from build123d import *

# Parameters (mm, degrees)
F0_W     = 42
F0_H     = 60
F0_R     = 5.1
F1_DEPTH = 25
F2_R     = 8.75
F2_R_2   = 5.1
F3_DEPTH = 35
F4_DEPTH = 60


with BuildPart() as f1:
    # F0 (on Top) → F1 (new body)
    with BuildSketch(Plane.XY):
        with Locations((-21, -12.544838)):
            Rectangle(F0_W, F0_H)
        with Locations((-12, 5.455162)):
            Circle(F0_R, mode=Mode.SUBTRACT)
    extrude(amount=F1_DEPTH)

    # F2 (on face) → F3 (cut)
    with BuildSketch(Plane(origin=(0, 17.455162, 0), x_dir=(-1, 0, 0), z_dir=(0, 1, 0))):
        with Locations((30, 12.5)):
            Circle(F2_R)
        with Locations((30, 12.5)):
            Circle(F2_R_2, mode=Mode.SUBTRACT)
    extrude(amount=-F3_DEPTH, mode=Mode.SUBTRACT)

    # F2 (on face) → F4 (cut)
    with BuildSketch(Plane(origin=(0, 17.455162, 0), x_dir=(-1, 0, 0), z_dir=(0, 1, 0))):
        with Locations((30, 12.5)):
            Circle(F2_R_2)
    extrude(amount=-F4_DEPTH, mode=Mode.SUBTRACT)


solid = f1.part
Could you check a few things on this model? Use its own coordinates, in mm. A direction names the side the tool comes from. Give positions to 0.01 mm unless a question says otherwise; leave off trailing zeros. Loops run counter-clockwise (first coordinate to the right, second up) from the corner with the lowest first, then second, coordinate; pieces in that order, holes last. Notation, with made-up numbers: M 11.5,42.25 L 54.5,42.25 A10 cw 54.5,61.25 Z; hole C -14,69 d8. An arc over 180 degrees is marked long. Answer as a JSON object with one key per item and string values.
Q1. If I drill on probe 1 along Z at (x, y) = (-30, -4); probe 2 along Y at (x, z) = (-12, 12.75); probe 3 along X at (y, z) = (9.5, 17.25), over which ranges is the centre line in solid material (lowest first)? Write a range as [from, to].
Values found:
{"probe 1": "z = [0, 3.75], [21.25, 25]", "probe 2": "y = [-42.54, 0.36], [10.56, 17.46]", "probe 3": "x = [-42, -37.35], [-22.65, -15.11], [-8.89, 0]"}
Q2. If we mould it in two halves opening along X, with no side actions, what happens to faces 1 (the flat face through (0, -13, 12)), 2 (the flat face through (-21, -42.545, 12)), 3 (the cylindrical face through (-7.29, 3.5, 12.32))? For each: pulls with the +X half, pulls with the -X half, needs draft (parallel to the pull), parting line crosses it, or undercut.
Values found:
{"face 1": "pulls with the +X half", "face 2": "needs draft", "face 3": "undercut"}
Q3. Suppose I cut it at A-A, the plane z = 12.5. List the corners of the cut face in (x, y) for me.
Values found:
{"outline": "M -42,-42.54 L -35.1,-42.54 L -35.1,-17.54 L -38.75,-17.54 L -38.75,17.46 L -42,17.46 Z; M -24.9,-42.54 L 0,-42.54 L 0,17.46 L -21.25,17.46 L -21.25,-17.54 L -24.9,-17.54 Z; hole C -12,5.46 d10.2"}
Q4. Suppose I cut it at C-C, the plane z = 20.5. List the corners of the cut face in (x, y) for me, plus the area to 3 significant figures.
Values found:
{"outline": "M -42,-42.54 L 0,-42.54 L 0,17.46 L -26.46,17.46 L -26.46,-17.54 L -33.54,-17.54 L -33.54,17.46 L -42,17.46 Z; hole C -12,5.46 d10.2", "area": "2,190 mm²"}
Q5. For faces 4 (the flat face through (-21, -12, 0)), 5 (the cylindrical face through (-28.861, 0.2, 21.176)), which set-ups out of +Z, -Z, +X, -X, +Y, -Y let a thin tool reach every point of the face, with its end or its side?
Values found:
{"face 4": "-Z, +X, -X, +Y, -Y", "face 5": "+Y"}
Q6. For P1, Ø14, axis at x = -30, z = 12.5, coming from the +Y side, with a flat end and sliding along its axis, tell me the tip position at first contact or that it passes through.
Values found:
{"P1": "stops at y = -17.54"}
Q7. Suppose I cut it at D-D, the plane y = -21. List the corners of the cut face in (x, z) for me, plus the area to 3 significant figures.
Values found:
{"outline": "M -42,0 L 0,0 L 0,25 L -42,25 Z; hole C -30,12.5 d10.2", "area": "968 mm²"}
Q8. Suppose I cut it at B-B, the plane x = -12. List the corners of the cut face in (y, z) for me, plus the area to 4 significant figures.
Values found:
{"outline": "M -42.54,0 L 0.36,0 L 0.36,25 L -42.54,25 Z; M 10.56,0 L 17.46,0 L 17.46,25 L 10.56,25 Z", "area": "1,245 mm²"}
